```python
from build123d import *

# Parameters (mm, degrees)
SKETCH_1_W           = 31.4
SKETCH_1_H           = 10
SKETCH_1_H_2         = 3
EXTRUDE_1_DEPTH      = 5
SKETCH_2_W           = 3.1
SKETCH_2_H           = 3.8
CUT_EXTRUDE_1_DEPTH  = 6
SKETCH_3_R           = 1.5
EXTRUDE_2_DEPTH      = 20.2
EXTRUDE_2_DEPTH_BACK = 20.2
SKETCH_5_W           = 9.55
SKETCH_5_H           = 3.6506089
SKETCH_5_W_2         = 12.3
SKETCH_5_H_2         = 6.45906725
CUT_EXTRUDE_2_DEPTH  = 5
SKETCH_6_R           = 0.75
CUT_EXTRUDE_3_DEPTH  = 41.4


with BuildPart() as part:
    # 草图1 → 凸台-拉伸1 (new body)
    with BuildSketch(Plane.XY):
        Rectangle(SKETCH_1_W, SKETCH_1_H)
        with Locations((0, 6.5)):
            Rectangle(SKETCH_1_W, SKETCH_1_H_2)
        Polygon((-15.7, 8), (-20.2, 8), (-15.7, -2.2), (-15.7, 5), align=None)
        Polygon((20.2, 8), (15.7, 8), (15.7, 5), (15.7, -2.2), align=None)
    extrude(amount=EXTRUDE_1_DEPTH)

    # 草图2 → 切除-拉伸1 (cut, through all)
    with BuildSketch(Plane.XY.offset(5)):
        with Locations((-13.05, 1.6)):
            Rectangle(SKETCH_2_W, SKETCH_2_H)
        with Locations((13.05, 1.6)):
            Rectangle(SKETCH_2_W, SKETCH_2_H)
    extrude(amount=-CUT_EXTRUDE_1_DEPTH, mode=Mode.SUBTRACT)

    # 草图3 → 凸台-拉伸2 (add, two sides)
    with BuildSketch(Plane(origin=(0, 0, 0), x_dir=(0, 0, -1), z_dir=(1, 0, 0))) as extrude_2_sk:
        with Locations((-2.5, 8)):
            Circle(SKETCH_3_R)
    extrude(amount=EXTRUDE_2_DEPTH)
    extrude(extrude_2_sk.sketch, amount=-EXTRUDE_2_DEPTH_BACK)

    # 草图5 → 切除-拉伸2 (cut)
    with BuildSketch(Plane.XY.offset(5)):
        with Locations((-10.925, 8)):
            Rectangle(SKETCH_5_W, SKETCH_5_H)
        with Locations((10.925, 8)):
            Rectangle(SKETCH_5_W, SKETCH_5_H)
        with Locations((0, -5)):
            Rectangle(SKETCH_5_W_2, SKETCH_5_H_2)
    extrude(amount=-CUT_EXTRUDE_2_DEPTH, mode=Mode.SUBTRACT)

    # 草图6 → 切除-拉伸3 (cut, through all)
    with BuildSketch(Plane.ZY.offset(20.2)):
        with Locations((2.5, 8)):
            Circle(SKETCH_6_R)
        with Locations((2.5, -3.8)):
            Circle(SKETCH_6_R)
    extrude(amount=-CUT_EXTRUDE_3_DEPTH, mode=Mode.SUBTRACT)


solid = part.part
```
Design review of the part built by this model. Coordinates are the model's own, in mm. A direction names the side the tool comes from. Coordinates: 2 decimals unless noted, no trailing zeros. Order: outer loops, then holes, each group sorted by start corner. A loop starts at its lowest first (then second) coordinate and runs counter-clockwise, first axis right, second up. Notation, with made-up numbers: M -7.75,88 L 17.25,88 A27 cw 17.25,115 Z; hole C 0,0.5 d4. An arc over 180 degrees is marked long. Answer as a JSON object with one key per item and string values. Group by question number.
1) Add section D-D, the plane z = 2.5. Count the separate pieces of the cut face and the enclosed holes in it, then the cut area to 3 significant figures.
2) Add section A-A, the plane x = 12. Write out the cut boundary in (y, z), then the cut area to 3 significant figures.
3) Add section B-B, the plane y = -3.8. Write out the cut boundary in (x, z), then the cut area to 4 significant figures.
4) Wall thickness on L1, parallel to Y at x = -12.5, z = 2.5; L2, parallel to Y at x = 14.5, z = 1.1; L3, parallel to Y at x = 9.25, z = 2.5: over which ranges is each line inside the solid? List them lowest first.
5) Tool access review of faces 5 (the flat face through (6.15, -3, 3)), 6 (the flat face through (-6.15, 7, 3)), 7 (the flat face through (14.6, 2, 3)), 8 (the flat face through (0.1, 8, 4.5)), 9 (the flat face through (0.1, 8, 0.5)): name each direction out of +Z, -Z, +X, -X, +Y, -Y from which nothing blocks a thin tool from reaching the whole face with its end or side.
6) For pin 1 (0.8 mm diameter, centred on x = -2.5, z = 0.5, fed in from +Y); pin 2 (2 mm diameter, centred on y = -3.8, z = 2.5, fed in from +X); pin 3 (1.5 mm diameter, centred on x = 10.5, z = 1.5, fed in from +Y), all flat-tipped, find the tip position at first contact; note any pin that passes through.
7) Add section C-C, the plane x = 0.5. Write out the cut boundary in (y, z), then the cut area to 3 significant figures.
8) Mouldability with a two-part tool opening along Z and no side actions: class faces 1 (the cylindrical face through (-17.9, 9.5, 2.5)), 2 (the flat face through (0, 2, 5)), 3 (the cylindrical face through (17.92, 7.71, 3.19)), 4 (the flat face through (11, 6.175, 3)) as pulls with the +Z half, pulls with the -Z half, needs draft (parallel to the pull), parting line crosses it, or undercut.
Computed values:
{
 "1": {"separate pieces": "6", "enclosed holes": "2", "area": "328 mm^2"},
 "2": {"outline": "M -5,0 L -0.3,0 L -0.3,5 L -5,5 Z; M 3.5,0 L 6.17,0 L 6.17,5 L 3.5,5 Z; hole C -3.8,2.5 d1.5", "area": "35.1 mm^2"},
 "3": {"outline": "M -15.7,0 L -6.15,0 L -6.15,1.75 L -15.7,1.75 Z; M -15.7,3.25 L -6.15,3.25 L -6.15,5 L -15.7,5 Z; M 6.15,0 L 15.7,0 L 15.7,1.75 L 6.15,1.75 Z; M 6.15,3.25 L 15.7,3.25 L 15.7,5 L 6.15,5 Z", "area": "66.85 mm^2"},
 "4": {"L1": "y = -5 to -4.55, -3.05 to -0.3, 3.5 to 6.17", "L2": "y = -5 to -0.3, 3.5 to 6.17", "L3": "y = -5 to -4.55, -3.05 to 6.17"},
 "5": {"face 5": "+Z, -Z, -Y", "face 6": "+Z, -Z, +Y", "face 7": "+Z, -Z", "face 8": "+Z, +X, -X, +Y", "face 9": "-Z, +X, -X, +Y"},
 "6": {"pin 1": "stops at y = 8", "pin 2": "stops at x = 15.7", "pin 3": "stops at y = 6.17"},
 "7": {"outline": "M -1.77,0 L 8,0 L 8,1 A1.5 ccw 8,4 L 8,5 L -1.77,5 Z; hole C 8,2.5 d1.5", "area": "50.6 mm^2"},
 "8": {"face 1": "parting line crosses it", "face 2": "pulls with the +Z half", "face 3": "undercut", "face 4": "needs draft"}
}
